```python
from build123d import *

# Parameters (mm, degrees)
SKETCH1_W           = 53
SKETCH1_H           = 20
SKETCH1_R           = 3.4
SKETCH1_R_2         = 3
BOSS_EXTRUDE2_DEPTH = 7


with BuildPart() as part:
    # Sketch1 → Boss-Extrude2 (new body)
    with BuildSketch(Plane.XY):
        with Locations((-46.622487041, -17.128716042)):
            Rectangle(SKETCH1_W, SKETCH1_H)
        with Locations((-68.122487041, -15.128716042)):
            Circle(SKETCH1_R, mode=Mode.SUBTRACT)
        Polygon((-63.122487041, -19.628716042), (-63.122487041, -9.628716042), (-30.122487041, -9.628716042), (-30.122487041, -19.628716042), (-27.122487041, -19.628716042), (-27.122487041, -24.628716042), (-30.122487041, -24.628716042), (-63.122487041, -24.628716042), (-66.122487041, -24.628716042), (-66.122487041, -19.628716042), align=None, mode=Mode.SUBTRACT)
        with Locations((-25.122487041, -15.128716042)):
            Circle(SKETCH1_R_2, mode=Mode.SUBTRACT)
    extrude(amount=BOSS_EXTRUDE2_DEPTH)


solid = part.part
```
The model under review builds one solid part; all positions refer to its coordinate system, in mm. A direction names the side the tool comes from. Round coordinates to 2 decimals unless told otherwise and drop trailing zeros. Loops run counter-clockwise (first coordinate to the right, second up) from the corner with the lowest first, then second, coordinate; pieces in that order, holes last. Notation, with made-up numbers: M 45,-7.75 L 90,-7.75 A14 cw 90,13.25 Z; hole C 59.5,-23.75 d2. An arc over 180 degrees is marked long. Write item = value, one per line.
Item 1: Insertion check: P1, Ø4, axis at x = -68.12, y = -15.13, coming from the +Z side. The pin has a flat end and moves straight along its axis. Give the tip position at first contact, or say it passes through.
Return value:
P1 = through
Item 2: Machinability: for faces 1 (the flat face through (-20.122, -17, 3)), 2 (the flat face through (-30.122, -15, 3)), which of the approach directions +Z, -Z, +X, -X, +Y, -Y give a long, thin tool a straight path to every point of the face, cutting with its end or side? Answer none if there is none.
Return value:
face_1 = +Z, -Z, +X, +Y, -Y
face_2 = +Z, -Z
Item 3: The part is to be moulded in two halves that separate along Z. For faces 3 (the flat face through (-47, -8, 0)), 4 (the flat face through (-47, -8, 7)), 5 (the cylindrical face through (-22.26, -14.23, 3.45)), say which applies: released by +Z, released by -Z, zero draft, split by the parting line, or undercut.
Return value:
face_3 = released by -Z
face_4 = released by +Z
face_5 = zero draft
Item 4: Take a section at C-C on y = -13.5. Write out the cut boundary in (x, z), then the cut area to 3 significant figures.
Return value:
outline = M -73.12,0 L -71.11,0 L -71.11,7 L -73.12,7 Z; M -65.14,0 L -63.12,0 L -63.12,7 L -65.14,7 Z; M -30.12,0 L -27.64,0 L -27.64,7 L -30.12,7 Z; M -22.6,0 L -20.12,0 L -20.12,7 L -22.6,7 Z
area = 62.9 mm2
Item 5: Take a section at B-B on y = -11. Write out the cut boundary in (x, z), then the cut area to 3 significant figures.
Return value:
outline = M -73.12,0 L -63.12,0 L -63.12,7 L -73.12,7 Z; M -30.12,0 L -20.12,0 L -20.12,7 L -30.12,7 Z
area = 140 mm2
Item 6: For line 1 (Y direction, x = -48, z = 3.75); line 2 (X direction, y = -16, z = 6.25); line 3 (X direction, y = -20, z = 1.5), list the stretches that pass through material, from the lowest coordinate up. Write a range as [from, to].
Return value:
line_1 = [-27.13, -24.63], [-9.63, -7.13]
line_2 = [-73.12, -71.41], [-64.84, -63.12], [-30.12, -27.99], [-22.25, -20.12]
line_3 = [-73.12, -66.12], [-27.12, -20.12]
Item 7: Take a section at A-A on x = -57. Write out the cut boundary in (y, z).
Return value:
outline = M -27.13,0 L -24.63,0 L -24.63,7 L -27.13,7 Z; M -9.63,0 L -7.13,0 L -7.13,7 L -9.63,7 Z
Item 8: Take a section at D-D on z = 3.75. Write out the cut boundary in (x, y), then the cut area to 3 significant figures.
Return value:
outline = M -73.12,-27.13 L -20.12,-27.13 L -20.12,-7.13 L -73.12,-7.13 Z; hole C -68.12,-15.13 d6.8; hole M -66.12,-24.63 L -27.12,-24.63 L -27.12,-19.63 L -30.12,-19.63 L -30.12,-9.63 L -63.12,-9.63 L -63.12,-19.63 L -66.12,-19.63 Z; hole C -25.12,-15.13 d6
area = 470 mm2
